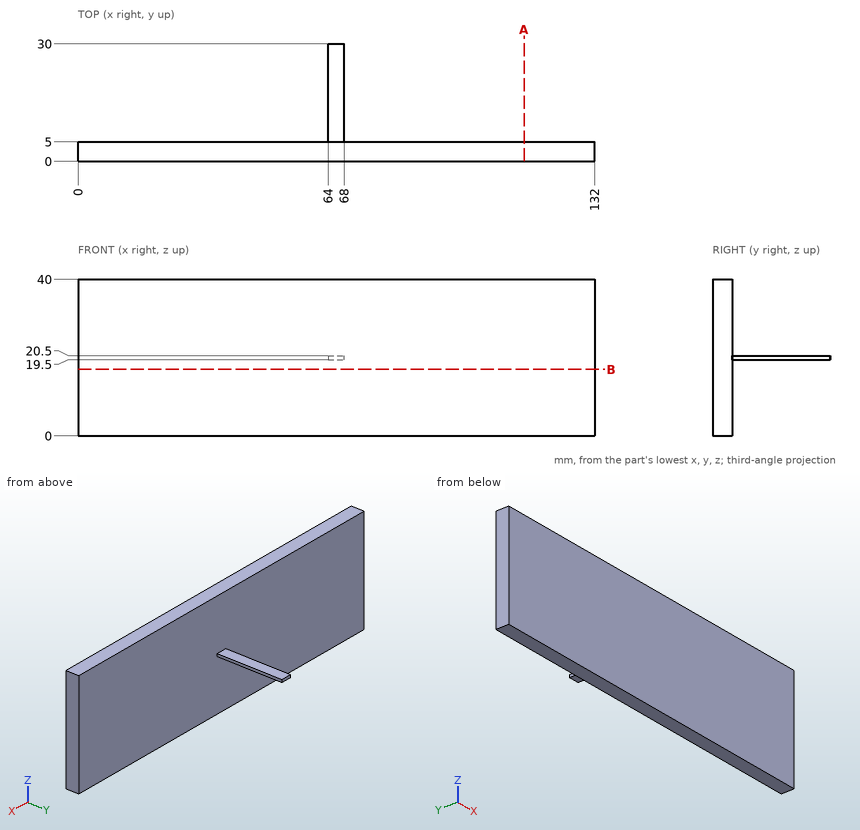
Geometry check sheet. Reference: drawing and pictorial views, mm from the part's lowest x, y, z. Round coordinates to 2 decimals unless told otherwise and drop trailing zeros. Loops run counter-clockwise (first coordinate to the right, second up) from the corner with the lowest first, then second, coordinate; pieces in that order, holes last. Notation, with made-up numbers: (-29, 77.5) - (8, 77.5) arc R21 cw to (8, 97.5) - close; hole circle Ø7 at (-3.5, 26). An arc over 180 degrees is marked (long way). Write item = value, one per line. Start each with the question number.
Q1. Depth check by flat-ended pin: P1, Ø4.5, axis at x = 67, y = 23.5, coming from the +Z side; P2, Ø6, axis at x = 24.5, z = 35.5, coming from the +Y side; P3, Ø1.5, axis at x = 40, y = 7, coming from the -Z side; P4, Ø12, axis at y = 15, z = 17, coming from the -X side. Enter the tip coordinate at first touch or a pass-through.
Q2. Section check B-B (z = 17). Record the boundary of the cut face in (x, y).
Q3. Section check A-A (x = 114). Record the boundary of the cut face in (y, z).
Q4. Thickness scan on L1, parallel to Y at x = 12, z = 15.5. Record the ranges inside material, lowest first.
Derived:
q1.P1 = 20.5
q1.P2 = 5
q1.P3 = through
q1.P4 = 64
q2.outline = (0, 0) - (132, 0) - (132, 5) - (0, 5) - close
q3.outline = (0, 0) - (5, 0) - (5, 40) - (0, 40) - close
q4.L1 = 0 to 5
